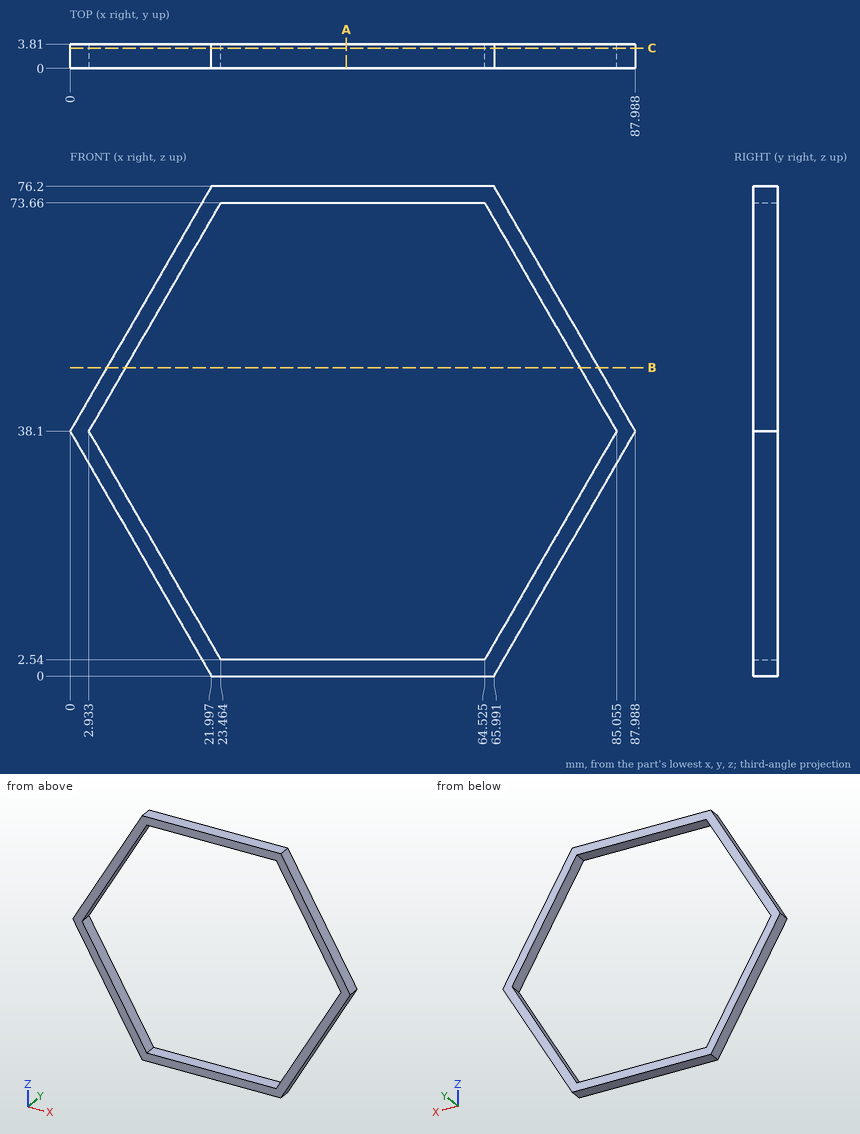
Design review of the part shown in the three views and the two pictorial views. Dimensions are in mm from the part's minimum x, y and z. Give positions to 0.01 mm unless a question says otherwise; leave off trailing zeros. Write each loop counter-clockwise with the first axis right and the second up, starting at its lowest first coordinate (ties: lowest second). Pieces come first, ordered by that corner, then holes. Notation, with made-up numbers: (86.5, 32) -> (132.5, 32) arc R15 ccw to (132.5, 61) -> close; hole circle Ø1 at (57.5, -25). An arc over 180 degrees is marked (long way). Answer in a Markdown table with one row per item.
1) For L1, parallel to Z at x = 51, y = 3.6; L2, parallel to X at y = 2.4, z = 55; L3, parallel to X at y = 0.7, z = 71.5 (1 decimal), list the stretches that pass through material, from the lowest coordinate up. Write a range as [from, to].
Worked answers:
| item | result |
|---|---|
| L1 | [0, 2.54], [73.66, 76.2] |
| L2 | [9.76, 12.69], [75.3, 78.23] |
| L3 | [19.3, 22.2], [65.8, 68.7] |
2) Add section C-C on y = 3.15. State the section outline as (x, z) points (1 decimal).
Worked answers:
| item | result |
|---|---|
| outline | (0, 38.1) -> (22, 0) -> (66, 0) -> (88, 38.1) -> (66, 76.2) -> (22, 76.2) -> close; hole (2.9, 38.1) -> (23.5, 2.5) -> (64.5, 2.5) -> (85.1, 38.1) -> (64.5, 73.7) -> (23.5, 73.7) -> close |
3) Add section B-B on z = 48. State the section outline as (x, y) points (1 decimal).
Worked answers:
| item | result |
|---|---|
| outline | (5.7, 0) -> (8.6, 0) -> (8.6, 3.8) -> (5.7, 3.8) -> close; (79.3, 0) -> (82.3, 0) -> (82.3, 3.8) -> (79.3, 3.8) -> close |
4) Add section A-A on x = 43. State the section outline as (y, z) points.
Worked answers:
| item | result |
|---|---|
| outline | (0, 0) -> (3.81, 0) -> (3.81, 2.54) -> (0, 2.54) -> close; (0, 73.66) -> (3.81, 73.66) -> (3.81, 76.2) -> (0, 76.2) -> close |
5) Clearance check with a flat-ended pin moving along its axis: P1, Ø1.5, axis at y = 1, z = 30, coming from the +X side (1 decimal). State where the tip first meets the part, or that it passes through.
Worked answers:
| item | result |
|---|---|
| P1 | x = 83.7 |
